from build123d import *

# Parameters (mm, degrees)
SKETCH1_R               = 12.5
BOSS_EXTRUDE1_DEPTH     = 14
SKETCH2_R               = 10
BOSS_EXTRUDE2_DEPTH     = 2
SKETCH3_R               = 12.5
BOSS_EXTRUDE3_DEPTH     = 30
SKETCH4_R               = 11.938790889
CUT_EXTRUDE1_DEPTH      = 1
SKETCH5_R               = 3.938949389
BOSS_EXTRUDE4_DEPTH     = 1
FILLET1_R               = 1
FILLET2_R               = 1
FILLET3_R               = 1
SKETCH6_R               = 1
CUT_EXTRUDE2_DEPTH      = 5
SKETCH7_R               = 4.25
BOSS_EXTRUDE5_DEPTH     = 3
FILLET4_R               = 0.5
SKETCH8_R               = 2
BOSS_EXTRUDE6_DEPTH     = 12
CUT_EXTRUDE3_DEPTH      = 64.509841777
CUT_EXTRUDE3_DEPTH_BACK = 9


with BuildPart() as part:
    # Sketch1 → Boss-Extrude1 (new body)
    with BuildSketch(Plane.XY):
        Circle(SKETCH1_R)
    extrude(amount=BOSS_EXTRUDE1_DEPTH)

    # Sketch2 → Boss-Extrude2 (add)
    with BuildSketch(Plane.XY.offset(14)):
        Circle(SKETCH2_R)
    extrude(amount=BOSS_EXTRUDE2_DEPTH)

    # Sketch3 → Boss-Extrude3 (add)
    with BuildSketch(Plane.XY.offset(16)):
        Circle(SKETCH3_R)
    extrude(amount=BOSS_EXTRUDE3_DEPTH)

    # Sketch4 → Cut-Extrude1 (cut)
    with BuildSketch(Plane.XY.offset(46)):
        Circle(SKETCH4_R)
    extrude(amount=-CUT_EXTRUDE1_DEPTH, mode=Mode.SUBTRACT)

    # Sketch5 → Boss-Extrude4 (add)
    with BuildSketch(Plane.XY.offset(45)):
        Circle(SKETCH5_R)
    extrude(amount=BOSS_EXTRUDE4_DEPTH)

    # Fillet1
    fillet1_edges = [part.edges().sort_by_distance(p)[0] for p in [
        (-3.938949389, 0, 46),
    ]]
    fillet(fillet1_edges, radius=FILLET1_R - 0.0001)  # a hair under: the kernel refuses the full size

    # Fillet2
    fillet2_edges = [part.edges().sort_by_distance(p)[0] for p in [
        (-12.5, 0, 0),
    ]]
    fillet(fillet2_edges, radius=FILLET2_R)

    # Fillet3
    fillet3_edges = [part.edges().sort_by_distance(p)[0] for p in [
        (-12.5, 0, 16),
        (-10, 0, 16),
    ]]
    fillet(fillet3_edges, radius=FILLET3_R)

    # Sketch6 → Cut-Extrude2 (cut)
    with BuildSketch(Plane(origin=(0, 0, 0), x_dir=(-1, 0, 0), z_dir=(0, 0, -1))):
        with Locations((-9.5, 0)):
            Circle(SKETCH6_R)
        with Locations((9.5, 0)):
            Circle(SKETCH6_R)
    extrude(amount=-CUT_EXTRUDE2_DEPTH, mode=Mode.SUBTRACT)

    # Sketch7 → Boss-Extrude5 (add)
    with BuildSketch(Plane(origin=(0, 0, 0), x_dir=(-1, 0, 0), z_dir=(0, 0, -1))):
        with Locations(Location((0, -3, 0), (0, 0, 180))):
            Circle(SKETCH7_R)
    extrude(amount=BOSS_EXTRUDE5_DEPTH)

    # Fillet4
    fillet4_edges = [part.edges().sort_by_distance(p)[0] for p in [
        (-4.25, -3, -3),
    ]]
    fillet(fillet4_edges, radius=FILLET4_R)

    # Sketch8 → Boss-Extrude6 (add)
    with BuildSketch(Plane(origin=(0, 0, -3), x_dir=(-1, 0, 0), z_dir=(0, 0, -1))):
        with Locations((0, -3)):
            Circle(SKETCH8_R)
    extrude(amount=BOSS_EXTRUDE6_DEPTH)

    # Sketch9 → Cut-Extrude3 (cut, two sides: drawn at the far end of the back side and taken through both)
    with BuildSketch(Plane(origin=(0, 0, -15), x_dir=(-1, 0, 0), z_dir=(0, 0, -1)).offset(-CUT_EXTRUDE3_DEPTH_BACK)):
        Polygon((-53.075925999, -8.559326208), (-1.919066235, -2.436808394), (1.731963356, -1.999848545), (52.88882312, 4.122669269), (40.643787491, 106.436388797), (-65.320961628, 93.754393319), align=None)
    extrude(amount=CUT_EXTRUDE3_DEPTH + CUT_EXTRUDE3_DEPTH_BACK, mode=Mode.SUBTRACT)


solid = part.part
Input: part model. Units: mm. Frame: model coordinates. A direction names the side the tool comes from. Coordinates: 2 decimals unless noted, no trailing zeros. Order: outer loops, then holes, each group sorted by start corner. A loop starts at its lowest first (then second) coordinate and runs counter-clockwise, first axis right, second up. Notation, with made-up numbers: M 19.25,13 L 38.25,13 A16 cw 38.25,24 Z; hole C -2,48 d10. An arc over 180 degrees is marked long. Write item = value, one per line. Start each with the question number.
(1) First-contact query: P1, Ø10, axis at x = -7, z = 15, coming from the -Y side; P2, Ø2.5, axis at x = 9.5, y = 0, coming from the +Z side; P3, Ø1.5, axis at y = 5.5, z = 12, coming from the +X side. Flat tips, straight axial feed; report the tip coordinate or a pass-through.
(2) Reachability of faces 5 (the flat face through (0.12, -2.22, -10.44)), 6 (the cylindrical face through (0, -5, -9)), 7 (the cylindrical face through (-9.474, -7.265, 45.507)), 8 (the flat face through (-0.1, 10.2, 14)) from +Z, -Z, +X, -X, +Y, -Y: full face, straight path, thin tool, end or side. Return the list, or none.
(3) Line query: line 1 along Y through (x, z) = (0, 45.3); line 2 along Z through (x, y) = (6, 0.25); line 3 along Z through (x, y) = (-7.75, -9). Output: solid intervals per line, ascending. Write a range as [from, to].
(4) Pull-direction query (X, two-part tool) for faces 1 (the cylindrical face through (-2.17, -9.76, 14.49)), 2 (the cylindrical face through (10.3, -0.6, 2.5)), 3 (the flat face through (0, 3, 0)), 4 (the flat face through (-3, 3, 45)); classes: released by +X, released by -X, zero draft, split by the parting line, or undercut.
(5) Section B-B on z = 37.5. Output: boundary loops of the cut face in (x, y).
(6) Section A-A on z = -10. Output: boundary loops of the cut face in (x, y).
Result set:
q1.P1 = -12.32
q1.P2 = 45
q1.P3 = 11.56
q2.face_5 = -Z, +X, +Y
q2.face_6 = -Z
q2.face_7 = +Z
q2.face_8 = none
q3.line_1 = [-12.5, -11.94], [-3.89, 3.89], [11.94, 12.5]
q3.line_2 = [0, 45]
q3.line_3 = [0.07, 14], [16.07, 45]
q4.face_1 = split by the parting line
q4.face_2 = undercut
q4.face_3 = zero draft
q4.face_4 = undercut
q5.outline = C 0,0 d25
q6.outline = M -1.73,-2 A2 ccw long 1.92,-2.44 Z
